Here's how the part is built. I have some questions about the finished solid (model axes, mm). A direction names the side the tool comes from. Round coordinates to 2 decimals unless told otherwise and drop trailing zeros. Write each loop counter-clockwise with the first axis right and the second up, starting at its lowest first coordinate (ties: lowest second). Pieces come first, ordered by that corner, then holes. Notation, with made-up numbers: (28.25, 34) - (69.25, 34) arc R6 ccw to (69.25, 42) - close; hole circle Ø10 at (27.25, 43.25). An arc over 180 degrees is marked (long way). Write item = value, one per line. Start each with the question number.
Item 1: Which directions (+Z, -Z, +X, -X, +Y, -Y) give clear straight access to the entire face, cutting with the end or side of a thin tool? Please do faces 1 (the face through (-0.1, -3.1, 50)), 2 (the face through (-4.1, 0, -24)), 3 (the face through (10.2, 0, 36)), 4 (the face through (12, 0, 30.07)).
Item 2: If we section it at C-C (x = -0.5): Please give me the cut outline in (y, z).
Item 3: If we section it at D-D (z = 11.5): Please give me the cut outline in (x, y), and give its area (3 significant figures).
Item 4: If we section it at A-A (z = 32): Please give me the cut outline in (x, y), and give its area (3 significant figures).
Item 5: If I drill on line 1 along X through (y, z) = (3.5, 32); line 2 along Z through (x, y) = (9.25, -1); line 3 along X through (y, z) = (0.5, -33.5), over which ranges is the centre line in solid material (lowest first)? Write a range as [from, to].
Item 6: Thinking about a two-plate mould opening in X: for faces 5 (the face through (14.2, 0, 42)), 6 (the face through (-10.2, 0, 36)), 7 (the face through (-12, 0, 30.07)), 8 (the face through (9, 0, 41.7)), which applies, pulls with the +X half, pulls with the -X half, needs draft (parallel to the pull), parting line crosses it, or undercut?
Item 7: For P1, Ø0.9, axis at x = -8, y = -0.5, coming from the -Z side; P2, Ø3, axis at x = 11, y = 1.5, coming from the -Z side; P3, Ø2, axis at y = 1, z = 7.5, coming from the -X side, each with a flat end and sliding along its axis, tell me the tip position at first contact or that it passes through.
```python
from build123d import *

# Parameters (mm, degrees)
F0_W     = 14.4
F0_H     = 100
F1_DEPTH = 4.5
F2_W     = 8.2
F2_H     = 5.7
F3_DEPTH = 100.001
F4_W     = 9
F4_H     = 1.3
F5_DEPTH = 6
F7_DEPTH = 9
F9_DEPTH = 50


with BuildPart() as f1:
    # F0 (on Front) → F1 (new body, symmetric)
    with BuildSketch(Plane.XZ):
        Rectangle(F0_W, F0_H)
    extrude(amount=F1_DEPTH, both=True)

    # F2 (on face) → F3 (cut, through all)
    with BuildSketch(Plane.XY.offset(50)):
        Rectangle(F2_W, F2_H)
    extrude(amount=-F3_DEPTH, mode=Mode.SUBTRACT)

    # F4 (on face) → F5 (join)
    with BuildSketch(Plane(origin=(-7.2, 0, 0), x_dir=(0, -1, 0), z_dir=(-1, 0, 0))):
        with Locations((0, 42.35)):
            Rectangle(F4_W, F4_H)
    extrude(amount=F5_DEPTH)

    # F6 (on face) → F7 (join)
    with BuildSketch(Plane(origin=(0, 4.5, 0), x_dir=(-1, 0, 0), z_dir=(0, 1, 0))):
        Polygon((10.2, 50.5525747299), (10.2, 30.0701190412), (14.2, 30.0701190412), (14.2, 53.9525747299), (10.2, 53.9525747299), align=None)
        Polygon((3.4, 50.5525747299), (10.2, 50.5525747299), (10.2, 53.9525747299), (3.4, 53.9525747299), (2.2, 53.9525747299), (2.2, 52.7525747299), align=None)
    extrude(amount=-F7_DEPTH)

    # F8: F1 across plane


with BuildPart() as f1_1:
    add(f1.part)
    add(f1.part.mirror(Plane.YZ))

    # F9 (add): a face of the model
    f9_faces = [f1_1.faces().sort_by_distance(p)[0] for p in [
        (-7.0301883396, 0, -50),
    ]]
    extrude(f9_faces, amount=F9_DEPTH)


solid = f1_1.part
```
Reply:
q1.face_1 = +Y, -Y
q1.face_2 = -Z
q1.face_3 = -Z, +Y, -Y
q1.face_4 = -Z, +X, +Y, -Y
q2.outline = (-4.5, -100) - (-2.85, -100) - (-2.85, 50) - (-4.5, 50) - close; (2.85, -100) - (4.5, -100) - (4.5, 50) - (2.85, 50) - close
q3.outline = (-7.2, -4.5) - (7.2, -4.5) - (7.2, 4.5) - (-7.2, 4.5) - close; hole (-4.1, -2.85) - (4.1, -2.85) - (4.1, 2.85) - (-4.1, 2.85) - close
q3.area = 82.9 mm2
q4.outline = (-14.2, -4.5) - (-10.2, -4.5) - (-10.2, 4.5) - (-14.2, 4.5) - close; (-7.2, -4.5) - (7.2, -4.5) - (7.2, 4.5) - (-7.2, 4.5) - close; (10.2, -4.5) - (14.2, -4.5) - (14.2, 4.5) - (10.2, 4.5) - close; hole (-4.1, -2.85) - (4.1, -2.85) - (4.1, 2.85) - (-4.1, 2.85) - close
q4.area = 155 mm2
q5.line_1 = [-14.2, -10.2], [-7.2, 7.2], [10.2, 14.2]
q5.line_2 = [41.7, 43], [50.55, 53.95]
q5.line_3 = [-7.2, -4.1], [4.1, 7.2]
q6.face_5 = pulls with the +X half
q6.face_6 = undercut
q6.face_7 = needs draft
q6.face_8 = undercut
q7.P1 = 41.7
q7.P2 = 30.07
q7.P3 = -7.2
